from build123d import *

# Parameters (mm, degrees)
SKETCH1_W           = 20
SKETCH1_H           = 100
SKETCH1_R           = 3
BOSS_EXTRUDE1_DEPTH = 10


with BuildPart() as part:
    # Sketch1 → Boss-Extrude1 (new body)
    with BuildSketch(Plane(origin=(0, 0, 0), x_dir=(1, 0, 0), z_dir=(0, 1, 0))):
        Rectangle(SKETCH1_W, SKETCH1_H)
        with Locations(Location((0, 45, 0), (0, 0, 270))):
            Circle(SKETCH1_R, mode=Mode.SUBTRACT)
        with BuildLine():
            Line((-3.25, 24), (-3.25, 26))
            ThreePointArc((-3.25, 26), (0, 29.25), (3.25, 26))
            Line((3.25, 26), (3.25, 24))
            ThreePointArc((3.25, 24), (0, 20.75), (-3.25, 24))
        make_face(mode=Mode.SUBTRACT)
        with BuildLine():
            Line((-3.25, -36), (-3.25, -34))
            ThreePointArc((-3.25, -34), (0, -30.75), (3.25, -34))
            Line((3.25, -34), (3.25, -36))
            ThreePointArc((3.25, -36), (0, -39.25), (-3.25, -36))
        make_face(mode=Mode.SUBTRACT)
    extrude(amount=BOSS_EXTRUDE1_DEPTH)


solid = part.part
The model under review builds one solid part; all positions refer to its coordinate system, in mm. A direction names the side the tool comes from. Coordinates: 2 decimals unless noted, no trailing zeros. Loops run counter-clockwise (first coordinate to the right, second up) from the corner with the lowest first, then second, coordinate; pieces in that order, holes last.
(1) Draft analysis for pull direction Z (two halves, no side actions). For faces 1 (the flat face through (-10, 5, 1)), 2 (the cylindrical face through (0, 5, -48)), 3 (the flat face through (0, 5, 50)), state which applies: +Z half, -Z half, draft (parallel to the pull), parting line (faces both ways), or undercut.
Determined:
face 1: draft
face 2: undercut
face 3: +Z half
(2) Consider section B-B, the plane y = 6.5. Give the boundary of the cut face in (x, z), plus the area to 3 significant figures.
Determined:
outline: (-10, -50) - (10, -50) - (10, 50) - (-10, 50) - close; hole (-3.25, -26) arc R3.25 ccw to (3.25, -26) - (3.25, -24) arc R3.25 ccw to (-3.25, -24) - close; hole (-3.25, 34) arc R3.25 ccw to (3.25, 34) - (3.25, 36) arc R3.25 ccw to (-3.25, 36) - close; hole circle Ø6 at (0, -45)
area: 1,880 mm2
(3) Consider section D-D, the plane z = 32. Give the boundary of the cut face in (x, y).
Determined:
outline: (-10, 0) - (-2.56, 0) - (-2.56, 10) - (-10, 10) - close; (2.56, 0) - (10, 0) - (10, 10) - (2.56, 10) - close
(4) Tool access review of faces 4 (the flat face through (0, 5, -50)), 5 (the flat face through (3.25, 5, -25)): name each direction out of +Z, -Z, +X, -X, +Y, -Y from which nothing blocks a thin tool from reaching the whole face with its end or side.
Determined:
face 4: -Z, +X, -X, +Y, -Y
face 5: +Y, -Y
(5) Wall thickness on L1, parallel to X at y = 7.75, z = -24; L2, parallel to X at y = 5, z = -45; L3, parallel to Z at x = -2, y = 3.75: over which ranges is each line inside the solid? List them lowest first.
Determined:
L1: x = -10 to -3.25, 3.25 to 10
L2: x = -10 to -3, 3 to 10
L3: z = -50 to -47.24, -42.76 to -28.56, -21.44 to 31.44, 38.56 to 50
(6) Consider section C-C, the plane x = 0. Give the boundary of the cut face in (y, z).
Determined:
outline: (0, -50) - (10, -50) - (10, -48) - (0, -48) - close; (0, -42) - (10, -42) - (10, -29.25) - (0, -29.25) - close; (0, -20.75) - (10, -20.75) - (10, 30.75) - (0, 30.75) - close; (0, 39.25) - (10, 39.25) - (10, 50) - (0, 50) - close
(7) Consider section A-A, the plane z = -45. Give the boundary of the cut face in (x, y), plus the area to 3 significant figures.
Determined:
outline: (-10, 0) - (-3, 0) - (-3, 10) - (-10, 10) - close; (3, 0) - (10, 0) - (10, 10) - (3, 10) - close
area: 140 mm2
